Autodesk Fusion 360 part; units mm, degrees
sketch "Esquisse1" plane through (0, 0, 0) normal (0, 0, 1) x (1, 0, 0)
  line L0 (75, 10) -> (-75, 10)
  line L1 (-75, 10) -> (-75, -10)
  line L2 (-75, -10) -> (75, -10)
  line L3 (75, -10) -> (75, 10)
  line L4 (75, 10) -> (-75, -10) construction
  line L5 (-75, 10) -> (75, -10) construction
  line L6 (-5, 10) -> (0, 10)
  line L7 (0, 10) -> (0, 15)
  line L8 (0, 15) -> (-5, 15)
  line L9 (-5, 15) -> (-5, 10)
  line L10 (-5, -10) -> (0, -10)
  line L11 (0, -10) -> (0, -15)
  line L12 (0, -15) -> (-5, -15)
  line L13 (-5, -15) -> (-5, -10)
  circle A0 centre (64.8598, 0) radius 7.5
  dimension "d1" = 150
  dimension "d2" = 20
  dimension "d3" = 5
  dimension "d4" = 5
  dimension "d5" = 70
  dimension "d6" = 5
  dimension "d7" = 5
  dimension "d8" = 15
  dimension "d35" = 70
extrude "Extrusion1" add sketch "Esquisse1" along normal blind 15
extrude "Extrusion2" cut sketch "Esquisse1" along normal blind 6 contours L0 L6 L7 L8 L9 | L2 L10 L11 L12 L13
fillet "Congé1" radius 5 4 edges at (-75, 10, 7.5) (-75, -10, 7.5) (75, 10, 7.5) (75, -10, 7.5)
extrude "Extrusion3" cut sketch "Esquisse1" along normal blind 3 contours L0 L1 L2 L3 L6 L10
extrude "Extrusion4" cut 2 faces at (-3.3333, -11.6667, 6) (-1.6667, 11.6667, 6) along direction (0, 0, 1) blind 4
fillet "Congé2" radius 1 4 edges at (-5, -15, 12.5) (0, -15, 12.5) (-5, 15, 12.5) (0, 15, 12.5)
extrude "Extrusion5" add sketch "Esquisse1" along normal blind 30 contours A0
extrude "Extrusion6" cut sketch "Esquisse1" along normal blind 3 contours A0
fillet "Congé3" radius 7 1 edges at (57.8673, -2.7121, 30)
extrude "Extrusion7" cut 1 faces at (23.3333, -3.3333, 3) along direction (0, 0, 1) blind 5
extrude "Extrusion8" cut 1 faces at (23.3333, -3.3333, 8) along direction (0, 0, 1) blind 1
extrude "Extrusion9" cut 2 faces at (-3.3333, -11.3333, 10) (-3.3333, 11.3333, 10) along direction (0, 0, 1) blind 3
extrude "Extrusion10" cut 1 faces at (23.3333, -3.3333, 9) along direction (0, 0, 1) blind 1
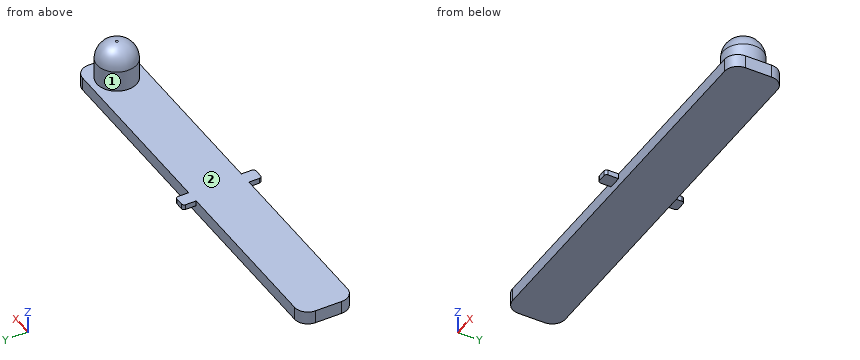
Source: CAD feature listing. Evaluate the final solid. Frame: model axes, mm. Face numbers are marked on the shaded views. Coordinates: 2 decimals unless noted, no trailing zeros. Loops run counter-clockwise (first coordinate to the right, second up) from the corner with the lowest first, then second, coordinate; pieces in that order, holes last. Notation, with made-up numbers: (53, 19.5) - (111, 19.5) arc R20 cw to (111, 28.5) - close; hole circle Ø10 at (18, 50.5). An arc over 180 degrees is marked (long way). One line per question, with ' | ' between items.
1) Pull-direction query (Y, two-part tool) for the marked faces 1 and 2; classes: released by +Y, released by -Y, zero draft, split by the parting line, or undercut.
Report:
face 1: split by the parting line | face 2: zero draft
2) Section B-B, the plane x = 55. Return loops of the section in (y, z), then the cut area to 3 significant figures.
Report:
outline: (-10, 10) - (10, 10) - (10, 15) - (-10, 15) - close | area: 100 mm²
3) Line query: line 1 along Z through (x, y) = (-46, 2.25); line 2 along X through (y, z) = (1.5, 15.75); line 3 along X through (y, z) = (-7.25, 13.5). Output: solid intervals per line, ascending.
Report:
line 1: z = 10 to 15 | line 2: x = 57.51 to 72.21 | line 3: x = -74.47 to 74.47
4) First-contact query: P1, Ø6, axis at x = -25, y = 3, coming from the +Z side; P2, Ø1.5, axis at x = 12.5, z = 12.5, coming from the -Y side; P3, Ø1, axis at x = 18, z = 13, coming from the +Y side. Flat tips, straight axial feed; report the tip coordinate or a pass-through.
Report:
P1: stops at z = 15 | P2: stops at y = -10 | P3: stops at y = 10
5) Section A-A, the plane z = 19.25. Return loops of the section in (x, y), then the cut area to 3 significant figures.
Report:
outline: circle Ø15 at (64.86, 0) | area: 177 mm²
